from build123d import *

# Parameters (mm, degrees)
TUBE_R            = 3.25
TUBE_R_2          = 1.25
TUBE_DEPTH        = 3.5
FILLET008_R       = 0.5
CYLINDER033_R     = 5
CYLINDER033_DEPTH = 2
FILLET007_R       = 1


with BuildPart() as fillet008:
    # Tube → Tube (new body)
    with BuildSketch(Plane(origin=(75.3, 6.35, 8.3), x_dir=(0, 0, -1), z_dir=(1, 0, 0))):
        Circle(TUBE_R)
        Circle(TUBE_R_2, mode=Mode.SUBTRACT)
    extrude(amount=TUBE_DEPTH)

    # Fillet008
    fillet008_edges = [fillet008.edges().sort_by_distance(p)[0] for p in [
        (75.3, 6.35, 11.55),
        (75.3, 6.35, 9.55),
    ]]
    fillet(fillet008_edges, radius=FILLET008_R)


with BuildPart() as dc_cap:
    # Cylinder033 → Cylinder033 (new body)
    with BuildSketch(Plane(origin=(78.8, 6.35, 8.3), x_dir=(0, 0, -1), z_dir=(1, 0, 0))):
        Circle(CYLINDER033_R)
    extrude(amount=CYLINDER033_DEPTH)

    # Fillet007
    fillet007_edges = [dc_cap.edges().sort_by_distance(p)[0] for p in [
        (80.8, 6.35, 13.3),
    ]]
    fillet(fillet007_edges, radius=FILLET007_R)

    # Fusion028: union Fillet008
    add(fillet008.part)


solid = dc_cap.part
Could you check a few things on this model? Use its own coordinates, in mm. A direction names the side the tool comes from. Coordinates: 2 decimals unless noted, no trailing zeros. Order: outer loops, then holes, each group sorted by start corner. A loop starts at its lowest first (then second) coordinate and runs counter-clockwise, first axis right, second up. Notation, with made-up numbers: (-25, 64) - (-15, 64) arc R16 cw to (-15, 86) - close; hole circle Ø4 at (-37, -35). An arc over 180 degrees is marked (long way). Answer in a Markdown table with one row per item. Add a question column.
(1) I need wall thicknesses on L1, parallel to Y at x = 76.9, z = 8.3; L2, parallel to X at y = 3, z = 7; L3, parallel to X at y = 6.5, z = 5.5. Which ranges of each line are inside material? Lowest first, please.
(2) Will these pins go through, and if not, where does the flat tip stop? pin 1 (1.5 mm diameter, centred on x = 77, z = 8.5, fed in from -Y); pin 2 (1 mm diameter, centred on x = 77, y = 8.5, fed in from -Z); pin 3 (2 mm diameter, centred on x = 76, z = 8, fed in from +Y).
(3) On a 3-axis mill with a long thin cutter (end or side, diameter ignored), from which of +Z, -Z, +X, -X, +Y, -Y can I reach the whole of each face in a straight line? I mean faces 1 (the face through (75.3, 8, 10)), 2 (the face through (78.8, 3, 7)). Say none if no direction works.
(4) If we section it at D-D, the plane x = 80.35: Please give me the cut outline in (y, z), then the cut area to 3 significant figures.
(5) If we section it at C-C, the plane x = 79.65: Please give me the cut outline in (y, z).
(6) If we section it at B-B, the plane y = 6.35: Please give me the cut outline in (x, z), then the cut area to 3 significant figures.
(7) If we section it at A-A, the plane z = 8.3: Please give me the cut outline in (x, y).
Results are:
| question | item | result |
|---|---|---|
| 1 | L1 | y = 3.1 to 5.1, 7.6 to 9.6 |
| 1 | L2 | x = 78.8 to 80.8 |
| 1 | L3 | x = 75.3 to 80.8 |
| 2 | pin 1 | stops at y = 3.1 |
| 2 | pin 2 | stops at z = 5.5 |
| 2 | pin 3 | stops at y = 9.6 |
| 3 | face 1 | +Z, -Z, -X, +Y, -Y |
| 3 | face 2 | -X |
| 4 | outline | circle Ø9.67 at (6.35, 8.3) |
| 4 | area | 73.4 mm2 |
| 5 | outline | circle Ø10 at (6.35, 8.3) |
| 6 | outline | (75.3, 5.55) arc R0.5 ccw to (75.8, 5.05) - (78.8, 5.05) - (78.8, 3.3) - (79.8, 3.3) arc R1 ccw to (80.8, 4.3) - (80.8, 12.3) arc R1 ccw to (79.8, 13.3) - (78.8, 13.3) - (78.8, 11.55) - (75.8, 11.55) arc R0.5 ccw to (75.3, 11.05) - (75.3, 10.05) arc R0.5 ccw to (75.8, 9.55) - (78.8, 9.55) - (78.8, 7.05) - (75.8, 7.05) arc R0.5 ccw to (75.3, 6.55) - close |
| 6 | area | 33.4 mm2 |
| 7 | outline | (75.3, 3.6) arc R0.5 ccw to (75.8, 3.1) - (78.8, 3.1) - (78.8, 1.35) - (79.8, 1.35) arc R1 ccw to (80.8, 2.35) - (80.8, 10.35) arc R1 ccw to (79.8, 11.35) - (78.8, 11.35) - (78.8, 9.6) - (75.8, 9.6) arc R0.5 ccw to (75.3, 9.1) - (75.3, 8.1) arc R0.5 ccw to (75.8, 7.6) - (78.8, 7.6) - (78.8, 5.1) - (75.8, 5.1) arc R0.5 ccw to (75.3, 4.6) - close |
